```python
from build123d import *

# Parameters (mm, degrees)
SKETCH_1_R      = 1.65
EXTRUDE_1_DEPTH = 2


with BuildPart() as part:
    # 草图1 → 凸台-拉伸1 (new body)
    with BuildSketch(Plane.XY):
        with BuildLine():
            ThreePointArc((3.478825803, 1.140085793), (31.160613474, 31.487300358), (22.098035111, 71.551055473))
            ThreePointArc((22.098035111, 71.551055473), (22.097226992, 71.552008754), (22.096419384, 71.552962467))
            ThreePointArc((22.096419384, 71.552962467), (24.398037137, 88.92818843), (41.467336112, 84.948872654))
            ThreePointArc((41.467336112, 84.948872654), (72.85197551, 66.494603701), (104.236614907, 84.948872654))
            ThreePointArc((104.236614907, 84.948872654), (121.305913882, 88.92818843), (123.607531636, 71.552962467))
            ThreePointArc((123.607531636, 71.552962467), (123.606724028, 71.552008754), (123.605915909, 71.551055473))
            ThreePointArc((123.605915909, 71.551055473), (114.543337545, 31.487300358), (142.225125217, 1.140085793))
            ThreePointArc((142.225125217, 1.140085793), (151.67398287, -12.372302839), (142.225125217, -25.884691472))
            ThreePointArc((142.225125217, -25.884691472), (114.543337545, -56.231906037), (123.605915909, -96.295661152))
            ThreePointArc((123.605915909, -96.295661152), (123.606724028, -96.296614433), (123.607531636, -96.297568146))
            ThreePointArc((123.607531636, -96.297568146), (121.305913882, -113.672794108), (104.236614907, -109.693478333))
            ThreePointArc((104.236614907, -109.693478333), (72.85197551, -91.23920938), (41.467336112, -109.693478333))
            ThreePointArc((41.467336112, -109.693478333), (24.398037137, -113.672794108), (22.096419384, -96.297568146))
            ThreePointArc((22.096419384, -96.297568146), (22.097226992, -96.296614433), (22.098035111, -96.295661152))
            ThreePointArc((22.098035111, -96.295661152), (31.160613474, -56.231906037), (3.478825803, -25.884691472))
            ThreePointArc((3.478825803, -25.884691472), (-5.97003185, -12.372302839), (3.478825803, 1.140085793))
        make_face()
        with Locations((11.842583941, -12.372302839)):
            Circle(SKETCH_1_R, mode=Mode.SUBTRACT)
        with Locations((119.681841833, 84.617416188)):
            Circle(SKETCH_1_R, mode=Mode.SUBTRACT)
        with Locations((36.414995742, 84.436007679)):
            Circle(SKETCH_1_R, mode=Mode.SUBTRACT)
        with Locations((36.233587233, 74.043121123)):
            Circle(SKETCH_1_R, mode=Mode.SUBTRACT)
        with Locations((4.492583941, -19.722302839)):
            Circle(SKETCH_1_R, mode=Mode.SUBTRACT)
        with Locations((114.57610281, 79.330268656)):
            Circle(SKETCH_1_R, mode=Mode.SUBTRACT)
        with Locations((119.863250342, 74.224529633)):
            Circle(SKETCH_1_R, mode=Mode.SUBTRACT)
        with Locations((141.211367078, -5.022302839)):
            Circle(SKETCH_1_R, mode=Mode.SUBTRACT)
        with Locations((109.470363787, 74.043121123)):
            Circle(SKETCH_1_R, mode=Mode.SUBTRACT)
        with Locations((148.561367078, -12.372302839)):
            Circle(SKETCH_1_R, mode=Mode.SUBTRACT)
        with Locations((141.211367078, -19.722302839)):
            Circle(SKETCH_1_R, mode=Mode.SUBTRACT)
        with Locations((141.211367078, -12.372302839)):
            Circle(SKETCH_1_R, mode=Mode.SUBTRACT)
        with Locations((109.288955277, 84.436007679)):
            Circle(SKETCH_1_R, mode=Mode.SUBTRACT)
        with Locations((133.861367078, -12.372302839)):
            Circle(SKETCH_1_R, mode=Mode.SUBTRACT)
        with Locations((4.492583941, -5.022302839)):
            Circle(SKETCH_1_R, mode=Mode.SUBTRACT)
        with Locations((26.022109187, -109.362021867)):
            Circle(SKETCH_1_R, mode=Mode.SUBTRACT)
        with Locations((31.12784821, -104.074874334)):
            Circle(SKETCH_1_R, mode=Mode.SUBTRACT)
        with Locations((25.840700677, -98.969135312)):
            Circle(SKETCH_1_R, mode=Mode.SUBTRACT)
        with Locations((25.840700677, 74.224529633)):
            Circle(SKETCH_1_R, mode=Mode.SUBTRACT)
        with Locations((31.12784821, 79.330268656)):
            Circle(SKETCH_1_R, mode=Mode.SUBTRACT)
        with Locations((26.022109187, 84.617416188)):
            Circle(SKETCH_1_R, mode=Mode.SUBTRACT)
        with Locations((109.288955277, -109.180613357)):
            Circle(SKETCH_1_R, mode=Mode.SUBTRACT)
        with Locations((109.470363787, -98.787726802)):
            Circle(SKETCH_1_R, mode=Mode.SUBTRACT)
        with Locations((119.863250342, -98.969135312)):
            Circle(SKETCH_1_R, mode=Mode.SUBTRACT)
        with Locations((114.57610281, -104.074874334)):
            Circle(SKETCH_1_R, mode=Mode.SUBTRACT)
        with Locations((36.233587233, -98.787726802)):
            Circle(SKETCH_1_R, mode=Mode.SUBTRACT)
        with Locations((36.414995742, -109.180613357)):
            Circle(SKETCH_1_R, mode=Mode.SUBTRACT)
        with Locations((119.681841833, -109.362021867)):
            Circle(SKETCH_1_R, mode=Mode.SUBTRACT)
        with Locations((-2.857416059, -12.372302839)):
            Circle(SKETCH_1_R, mode=Mode.SUBTRACT)
        with Locations((4.492583941, -12.372302839)):
            Circle(SKETCH_1_R, mode=Mode.SUBTRACT)
    extrude(amount=EXTRUDE_1_DEPTH)


solid = part.part
```
Work out the finished part from the listing and answer in its coordinate system (mm). Give positions to 0.01 mm unless a question says otherwise; leave off trailing zeros. Loops run counter-clockwise (first coordinate to the right, second up) from the corner with the lowest first, then second, coordinate; pieces in that order, holes last. Notation, with made-up numbers: M 84,-34 L 117,-34 A19 cw 117,-28 Z; hole C 87,-19 d6. An arc over 180 degrees is marked long. One line per item, written item: value. Start each with the question number.
1. Find section C-C (z = 0.3). State how many separate pieces and enclosed holes the cut face has, and give its area (3 significant figures).
2. Find the intervals of material crossed by probe 1 along X at (y, z) = (41.5, 0.1); probe 2 along X at (y, z) = (-5, 1.6); probe 3 along Y at (x, z) = (73, 0.7), in increasing order.
3. Find section A-A (y = 7). Give the vertices of the cut face in (x, z), and give its area (3 significant figures).
4. Determine the mould class of faces 1 (the face through (74, -11, 0)), 2 (the face through (151.67, -12.13, 0.99)), 3 (the face through (31, 30.9, 1)), 4 (the face through (121.08, 89.08, 0.99)) for opening direction X: released by +X, released by -X, zero draft, split by the parting line, or undercut.
5. Find section B-B (x = 79). Give the vertices of the cut face in (y, z).
Reported:
1. separate pieces: 1
1. enclosed holes: 30
1. area: 18,400 mm²
2. probe 1: x = 32.62 to 113.09
2. probe 2: x = -3.94 to 2.84, 6.14 to 139.56, 142.86 to 149.64
2. probe 3: y = -91.24 to 66.49
3. outline: M 14.44,0 L 131.26,0 L 131.26,2 L 14.44,2 Z
3. area: 234 mm²
4. face 1: zero draft
4. face 2: released by +X
4. face 3: released by -X
4. face 4: undercut
5. outline: M -91.77,0 L 67.02,0 L 67.02,2 L -91.77,2 Z
